The model under review builds one solid part; all positions refer to its coordinate system, in mm. A direction names the side the tool comes from. Give positions to 0.01 mm unless a question says otherwise; leave off trailing zeros. Loops run counter-clockwise (first coordinate to the right, second up) from the corner with the lowest first, then second, coordinate; pieces in that order, holes last. Notation, with made-up numbers: M -29.75,62.25 L 19.25,62.25 A37 ccw 19.25,100.25 Z; hole C 57,58.25 d11. An arc over 180 degrees is marked long. One line per item, written item: value. Start each with the question number.
Q1. Mouldability with a two-part tool opening along X and no side actions: class faces 1 (the face through (0, 6, 5)), 2 (the face through (17.352, 4, 7)), 3 (the face through (0.88, 39.99, -0.07)) as released by +X, released by -X, zero draft, split by the parting line, or undercut.
Q2. To check wall thickness, follow line 1 along Y through (x, z) = (0, -2.3); line 2 along Y through (x, z) = (0, 1.7); line 3 along X through (y, z) = (13, 7.75). State the ranges of each line that lie inside material, in increasing order. Write a range as from..to.
Q3. For faces 4 (the face through (13.89, 18.34, 6.97)), 5 (the face through (0.253, -18.594, 6.972)), 6 (the face through (-17.395, 4, 7)), 7 (the face through (12.069, 15.958, 6.972)), list the 3-axis set-ups (+Z, -Z, +X, -X, +Y, -Y) from which the entire face can be reached by the end or side of a thin tool; tool diameter is ignored.
Q4. For pin 1 (1.8 mm diameter, centred on x = 8.5, z = 6.5, fed in from -Y); pin 2 (1.2 mm diameter, centred on x = 4.5, z = 6.5, fed in from +Y); pin 3 (4 mm diameter, centred on x = 12.5, y = -33, fed in from +Z), all flat-tipped, find the tip position at first contact; note any pin that passes through.
Q5. We need section A-A on x = 0. Write out the cut boundary in (y, z), plus the area to 3 significant figures.
Q6. We need section B-B on z = 6.75. Write out the cut boundary in (x, y), plus the area to 3 significant figures.
Q7. We need section C-C on y = -47. Write out the cut boundary in (x, z), plus the area to 3 significant figures.
Q8. We need section D-D on z = -2. Write out the cut boundary in (x, y), plus the area to 3 significant figures.
```python
from build123d import *

# Parameters (mm, degrees)
SKETCH6_W           = 80
SKETCH6_H           = 106.2
BOSS_EXTRUDE3_DEPTH = 5
BOSS_EXTRUDE2_DEPTH = 4
CUT_EXTRUDE2_REACH  = 69.228
SKETCH4_R           = 4.5
SKETCH7_R           = 7.75
CUT_EXTRUDE3_DEPTH  = 5.5
CUT_EXTRUDE4_START  = -5
CUT_EXTRUDE4_DEPTH  = 10


with BuildPart() as part:
    # Sketch6 → Boss-Extrude3 (new, symmetric)
    with BuildSketch(Plane.XY):
        Rectangle(SKETCH6_W, SKETCH6_H)
    extrude(amount=BOSS_EXTRUDE3_DEPTH, both=True)

    # Sketch3 → Boss-Extrude2 (add)
    with BuildSketch(Plane.XY.offset(5)):
        with BuildLine():
            Line((-17.395287132, -6.571810208), (-17.395287132, 15.307157848))
            Line((-17.395287132, 15.307157848), (-15.311099774, 17.296395792))
            Line((-15.311099774, 17.296395792), (-12.46185448, 19.451424939))
            Line((-12.46185448, 19.451424939), (-10.63935497, 20.5))
            Line((-10.63935497, 20.5), (10.639354967, 20.5))
            Line((10.639354967, 20.5), (12.481546734, 19.440095002))
            Line((12.481546734, 19.440095002), (15.334663563, 17.215949154))
            Line((15.334663563, 17.215949154), (17.351649475, 15.287999429))
            Line((17.351649475, 15.287999429), (17.351649475, -6.686177108))
            ThreePointArc((17.351649475, -6.686177108), (-0.061204642, -18.595186415), (-17.395287132, -6.571810208))
        make_face()
        with BuildLine():
            Line((-14.395287132, -5.999057373), (-14.395287132, 14.02336094))
            Line((-14.395287132, 14.02336094), (-13.364210648, 15.007464628))
            Line((-13.364210648, 15.007464628), (-10.802429685, 16.945069879))
            Line((-10.802429685, 16.945069879), (-9.202356052, 17.865672216))
            Line((-9.202356052, 17.865672216), (-5.025287127, 17.865672216))
            Line((-5.025287127, 17.865672216), (-5.025287127, 18.307908255))
            ThreePointArc((-5.025287127, 18.307908255), (-4.850962964, 18.728764013), (-4.430107206, 18.903088176))
            Line((-4.430107206, 18.903088176), (6.970107208, 18.903088176))
            ThreePointArc((6.970107208, 18.903088176), (7.390962965, 18.728764013), (7.565287128, 18.307908255))
            Line((7.565287128, 18.307908255), (7.565287128, 17.865672216))
            Line((7.565287128, 17.865672216), (9.202356049, 17.865672216))
            Line((9.202356049, 17.865672216), (10.803064919, 16.944704398))
            Line((10.803064919, 16.944704398), (13.37101734, 14.942858327))
            Line((13.37101734, 14.942858327), (14.351649475, 14.00551442))
            Line((14.351649475, 14.00551442), (14.351649475, -6.102715652))
            ThreePointArc((14.351649475, -6.102715652), (-0.056234518, -15.595185752), (-14.395287132, -5.999057373))
        make_face(mode=Mode.SUBTRACT)
    extrude(amount=BOSS_EXTRUDE2_DEPTH)

    # Sketch4 → Cut-Extrude2 (cut, up to next)
    with BuildSketch(Plane.XY.offset(5), mode=Mode.PRIVATE) as cut_extrude2_sk1:
        Circle(SKETCH4_R)
    cut_extrude2_tool1 = extrude(cut_extrude2_sk1.sketch, amount=-CUT_EXTRUDE2_REACH, mode=Mode.PRIVATE) & part.part
    add(cut_extrude2_tool1.solids().sort_by_distance((0, 0, 5))[0], mode=Mode.SUBTRACT)

    # Sketch7 → Cut-Extrude3 (cut)
    with BuildSketch(Plane(origin=(0, 0, -5), x_dir=(-1, 0, 0), z_dir=(0, 0, -1))):
        Circle(SKETCH7_R)
    extrude(amount=-CUT_EXTRUDE3_DEPTH, mode=Mode.SUBTRACT)

    # Sketch8 → Cut-Extrude4 (cut)
    with BuildSketch(Plane.XY.offset(CUT_EXTRUDE4_START)):
        with BuildLine():
            Line((-40, 0), (-40, 53.1))
            Line((-40, 53.1), (40, 53.1))
            Line((40, 53.1), (40, 0))
            ThreePointArc((40, 0), (0, 40), (-40, 0))
        make_face()
    extrude(amount=CUT_EXTRUDE4_DEPTH, mode=Mode.SUBTRACT)


solid = part.part
```
Solved:
1. face 1: undercut
1. face 2: released by +X
1. face 3: split by the parting line
2. line 1: -53.1..-7.75, 7.75..40
2. line 2: -53.1..-4.5, 4.5..40
2. line 3: -17.4..-14.4, 14.35..17.35
3. face 4: +Z, +X, +Y
3. face 5: +Z, -Y
3. face 6: +Z, -X, +Y, -Y
3. face 7: +Z
4. pin 1: y = -16.97
4. pin 2: y = 20.5
4. pin 3: z = 5
5. outline: M -53.1,-5 L -7.75,-5 L -7.75,0.5 L -4.5,0.5 L -4.5,5 L -15.6,5 L -15.6,9 L -18.6,9 L -18.6,5 L -53.1,5 Z; M 4.5,0.5 L 7.75,0.5 L 7.75,-5 L 40,-5 L 40,5 L 20.5,5 L 20.5,9 L 18.9,9 L 18.9,5 L 4.5,5 Z
5. area: 824 mm2
6. outline: M -17.4,-6.57 A18.6 ccw 17.35,-6.69 L 17.35,15.29 L 15.33,17.22 L 12.48,19.44 L 10.64,20.5 L -10.64,20.5 L -12.46,19.45 L -15.31,17.3 L -17.4,15.31 Z; hole M -14.4,-6 A15.6 ccw 14.35,-6.1 L 14.35,14.01 L 13.37,14.94 L 10.8,16.94 L 9.2,17.87 L 7.57,17.87 L 7.57,18.31 A0.6 ccw 6.97,18.9 L -4.43,18.9 A0.6 ccw -5.03,18.31 L -5.03,17.87 L -9.2,17.87 L -10.8,16.95 L -13.36,15.01 L -14.4,14.02 Z
6. area: 333 mm2
7. outline: M -40,-5 L 40,-5 L 40,5 L -40,5 Z
7. area: 800 mm2
8. outline: M -40,-53.1 L 40,-53.1 L 40,0 A40 ccw -40,0 Z; hole C 0,0 d15.5
8. area: 6,570 mm2
